Work out the finished part from the listing and answer in its coordinate system (mm). Give positions to 0.01 mm unless a question says otherwise; leave off trailing zeros. Order: outer loops, then holes, each group sorted by start corner. A loop starts at its lowest first (then second) coordinate and runs counter-clockwise, first axis right, second up.
```python
from build123d import *

# Parameters (mm, degrees)
SKETCH1_W           = 300
SKETCH1_H           = 600
BOSS_EXTRUDE1_DEPTH = 3.175
CUT_EXTRUDE1_DEPTH  = 10
SKETCH4_R           = 2.05
CUT_EXTRUDE2_DEPTH  = 51
SKETCH5_R           = 2.1
CUT_EXTRUDE3_DEPTH  = 67
SKETCH7_R           = 2.05
CUT_EXTRUDE4_DEPTH  = 10
SKETCH8_R           = 2.1
CUT_EXTRUDE5_DEPTH  = 10


with BuildPart() as part:
    # Sketch1 → Boss-Extrude1 (new body)
    with BuildSketch(Plane(origin=(0, 0, 0), x_dir=(1, 0, 0), z_dir=(0, 1, 0))):
        Rectangle(SKETCH1_W, SKETCH1_H)
    extrude(amount=BOSS_EXTRUDE1_DEPTH)

    # Sketch3 → Cut-Extrude1 (cut)
    with BuildSketch(Plane(origin=(0, 3.175, 0), x_dir=(1, 0, 0), z_dir=(0, 1, 0))):
        with BuildLine():
            Line((-95, -255), (95, -255))
            ThreePointArc((95, -255), (102.071067812, -252.071067812), (105, -245))
            Line((105, -245), (105, 100))
            ThreePointArc((105, 100), (102.071067812, 107.071067812), (95, 110))
            Line((95, 110), (-95, 110))
            ThreePointArc((-95, 110), (-102.071067812, 107.071067812), (-105, 100))
            Line((-105, 100), (-105, -245))
            ThreePointArc((-105, -245), (-102.071067812, -252.071067812), (-95, -255))
        make_face()
        with BuildLine():
            Line((105, 255), (105, 165))
            ThreePointArc((105, 165), (102.071067812, 157.928932188), (95, 155))
            Line((95, 155), (-95, 155))
            ThreePointArc((-95, 155), (-102.071067992, 157.928932157), (-105.000000511, 165))
            Line((-105.000000511, 165), (-105.000005107, 255))
            Line((-105.000005107, 255), (-150, 255))
            Line((-150, 255), (-150, 300))
            Line((-150, 300), (150, 300))
            Line((150, 300), (150, 255))
            Line((150, 255), (105, 255))
        make_face()
    extrude(amount=-CUT_EXTRUDE1_DEPTH, mode=Mode.SUBTRACT)

    # Sketch4 → Cut-Extrude2 (cut)
    with BuildSketch(Plane(origin=(0, 3.175, 0), x_dir=(1, 0, 0), z_dir=(0, 1, 0))):
        with Locations((12, -291)):
            Circle(SKETCH4_R)
        with Locations((-12, -291)):
            Circle(SKETCH4_R)
        with Locations((-12, -278)):
            Circle(SKETCH4_R)
        with Locations((12, -278)):
            Circle(SKETCH4_R)
    extrude(amount=-CUT_EXTRUDE2_DEPTH, mode=Mode.SUBTRACT)

    # Sketch5 → Cut-Extrude3 (cut)
    with BuildSketch(Plane(origin=(0, 3.175, 0), x_dir=(1, 0, 0), z_dir=(0, 1, 0))):
        with Locations((137, -73.264775169)):
            Circle(SKETCH5_R)
        with Locations((137, -58.264775169)):
            Circle(SKETCH5_R)
    extrude(amount=-CUT_EXTRUDE3_DEPTH, mode=Mode.SUBTRACT)

    # Sketch7 → Cut-Extrude4 (cut)
    with BuildSketch(Plane(origin=(0, 3.175, 0), x_dir=(1, 0, 0), z_dir=(0, 1, 0))):
        with Locations((138.75, -288.75)):
            Circle(SKETCH7_R)
        with Locations((116.25, -266.25)):
            Circle(SKETCH7_R)
        with Locations((47.023601507, -266.25)):
            Circle(SKETCH7_R)
        with Locations((69.523601507, -288.75)):
            Circle(SKETCH7_R)
        with Locations((116.25, -171.25)):
            Circle(SKETCH7_R)
        with Locations((138.75, -193.75)):
            Circle(SKETCH7_R)
        with Locations((116.25, -76.25)):
            Circle(SKETCH7_R)
        with Locations((138.75, -98.75)):
            Circle(SKETCH7_R)
        with Locations((116.25, 18.75)):
            Circle(SKETCH7_R)
        with Locations((138.75, -3.75)):
            Circle(SKETCH7_R)
        with Locations((116.25, 113.75)):
            Circle(SKETCH7_R)
        with Locations((138.75, 91.25)):
            Circle(SKETCH7_R)
        with Locations((116.25, 208.75)):
            Circle(SKETCH7_R)
        with Locations((138.75, 186.25)):
            Circle(SKETCH7_R)
        with Locations((47.357849803, 121.25)):
            Circle(SKETCH7_R)
        with Locations((69.635017605, 143.75)):
            Circle(SKETCH7_R)
        with Locations((-47.357849803, 121.25)):
            Circle(SKETCH7_R)
        with Locations((-69.635017605, 143.75)):
            Circle(SKETCH7_R)
        with Locations((-116.25, 208.75)):
            Circle(SKETCH7_R)
        with Locations((-138.75, 186.25)):
            Circle(SKETCH7_R)
        with Locations((-138.75, 91.25)):
            Circle(SKETCH7_R)
        with Locations((-116.25, 18.75)):
            Circle(SKETCH7_R)
        with Locations((-116.25, 113.75)):
            Circle(SKETCH7_R)
        with Locations((-116.25, -76.25)):
            Circle(SKETCH7_R)
        with Locations((-138.75, -3.75)):
            Circle(SKETCH7_R)
        with Locations((-138.75, -98.75)):
            Circle(SKETCH7_R)
        with Locations((-116.25, -171.25)):
            Circle(SKETCH7_R)
        with Locations((-138.75, -193.75)):
            Circle(SKETCH7_R)
        with Locations((-116.25, -266.25)):
            Circle(SKETCH7_R)
        with Locations((-138.75, -288.75)):
            Circle(SKETCH7_R)
        with Locations((-47.023601507, -266.25)):
            Circle(SKETCH7_R)
        with Locations((-69.523601507, -288.75)):
            Circle(SKETCH7_R)
        with Locations((-138.75, 243.75)):
            Circle(SKETCH7_R)
        with Locations((138.75, 243.75)):
            Circle(SKETCH7_R)
    extrude(amount=-CUT_EXTRUDE4_DEPTH, mode=Mode.SUBTRACT)

    # Sketch8 → Cut-Extrude5 (cut)
    with BuildSketch(Plane(origin=(0, 3.175, 0), x_dir=(1, 0, 0), z_dir=(0, 1, 0))):
        with Locations((139.5, 210.665995932)):
            Circle(SKETCH8_R)
        with Locations((139.5, -244.701867271)):
            Circle(SKETCH8_R)
    cut_extrude5 = extrude(amount=-CUT_EXTRUDE5_DEPTH, mode=Mode.SUBTRACT)

    # Mirror1: Cut-Extrude5 across plane
    add(cut_extrude5.mirror(Plane(origin=(0, 0, 0), x_dir=(0, 0, 1), z_dir=(1, 0, 0))), mode=Mode.SUBTRACT)


solid = part.part
```
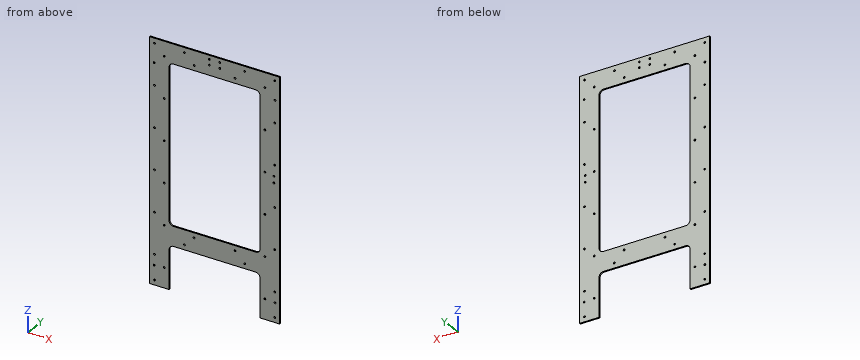
1. The part is cut by section A-A (z = 137). Write down the section's boundary in (x, y) (3 decimals), then the cut area to 3 significant figures.
Findings below:
outline: (-150, 0) - (-105, 0) - (-105, 3.175) - (-150, 3.175) - close; (105, 0) - (150, 0) - (150, 3.175) - (105, 3.175) - close
area: 286 mm2
2. Straight lines are drawn through the part: probe 1 along X at (y, z) = (2.5, 266.25); probe 2 along X at (y, z) = (2.3, -243.75); probe 3 along X at (y, z) = (2.15, -113.75). For each, find the intervals that lie inside material, in ascending order.
Findings below:
probe 1: x = -150 to -118.3, -114.2 to -49.07, -44.97 to 44.97, 49.07 to 114.2, 118.3 to 150
probe 2: x = -150 to -140.8, -136.7 to -105, 105 to 136.7, 140.8 to 150
probe 3: x = -150 to -118.3, -114.2 to 114.2, 118.3 to 150
3. The part is cut by section B-B (x = -78.5). Write down the section's boundary in (y, z) (3 decimals), then the cut area to 3 significant figures.
Findings below:
outline: (0, -155) - (3.175, -155) - (3.175, -110) - (0, -110) - close; (0, 255) - (3.175, 255) - (3.175, 300) - (0, 300) - close
area: 286 mm2
4. The part is cut by section C-C (y = 2.6). State how many separate pieces and enclosed holes the cut face has, then the cut area to 3 significant figures.
Findings below:
separate pieces: 1
enclosed holes: 45
area: 68,400 mm2
5. Given P1, Ø2.5, axis at x = 139.5, z = -210.67, coming from the -Y side, flat-ended and moving along its own axis, determine where the tip first touches the part or whether it passes through.
Findings below:
P1: passes through
